Source: CAD feature listing. Evaluate the final solid. Frame: model axes, mm. Give positions to 0.01 mm unless a question says otherwise; leave off trailing zeros. Loops run counter-clockwise (first coordinate to the right, second up) from the corner with the lowest first, then second, coordinate; pieces in that order, holes last. Notation, with made-up numbers: M -31,4 L 4,4 A28 ccw 4,23 Z; hole C -4,33 d3. An arc over 180 degrees is marked long. Put each result on its own line as item: value.
Autodesk Fusion 360 part; units mm, degrees
sketch "Boceto1" plane through (0, 0, 0) normal (0, 0, 1) x (1, 0, 0)
  circle A0 centre (0, 0) radius 2
  line L0 (-1.7321, 3) -> (-3.4641, 0)
  line L1 (-3.4641, 0) -> (-1.7321, -3)
  line L2 (-1.7321, -3) -> (1.7321, -3)
  line L3 (1.7321, -3) -> (3.4641, 0)
  line L4 (3.4641, 0) -> (1.7321, 3)
  line L5 (1.7321, 3) -> (-1.7321, 3)
  dimension "d1" = 4
extrude "Extruir1" add sketch "Boceto1" along normal blind 2
1. Draft query along Y for faces 1 (the cylindrical face through (0, 2, 1)), 2 (the flat face through (0, -3, 1)), 3 (the flat face through (1, 2, 2)). Return one class per face: pulls with the +Y half, pulls with the -Y half, needs draft (parallel to the pull), parting line crosses it, or undercut.
Found:
face 1: undercut
face 2: pulls with the -Y half
face 3: needs draft
2. Section query D-D (y = 2.3). Output: boundary loops of the cut face in (x, z), plus the area to 3 significant figures.
Found:
outline: M -2.14,0 L 2.14,0 L 2.14,2 L -2.14,2 Z
area: 8.54 mm^2
3. Section query C-C (y = -0.85). Output: boundary loops of the cut face in (x, z), plus the area to 3 significant figures.
Found:
outline: M -2.97,0 L -1.81,0 L -1.81,2 L -2.97,2 Z; M 1.81,0 L 2.97,0 L 2.97,2 L 1.81,2 Z
area: 4.65 mm^2
4. Material intervals for line 1 (Y direction, x = 0, z = 0.85); line 2 (X direction, y = -1.4, z = 1.2); line 3 (Y direction, x = -0.5, z = 1.85), sorted ascending. Write a range as from..to.
Found:
line 1: -3..-2, 2..3
line 2: -2.66..-1.43, 1.43..2.66
line 3: -3..-1.94, 1.94..3
5. Section query A-A (x = 0). Output: boundary loops of the cut face in (y, z).
Found:
outline: M -3,0 L -2,0 L -2,2 L -3,2 Z; M 2,0 L 3,0 L 3,2 L 2,2 Z
6. Section query B-B (z = 1.35). Output: boundary loops of the cut face in (x, y), plus the area to 3 significant figures.
Found:
outline: M -3.46,0 L -1.73,-3 L 1.73,-3 L 3.46,0 L 1.73,3 L -1.73,3 Z; hole C 0,0 d4
area: 18.6 mm^2
